Answer from the drawing. Dimensions are ordinates in mm from the lowest x, y and z of the part. A direction names the side the tool comes from. Coordinates: 2 decimals unless noted, no trailing zeros. Write each loop counter-clockwise with the first axis right and the second up, starting at its lowest first coordinate (ties: lowest second). Pieces come first, ordered by that corner, then holes.
(1) The part is cut by section B-B, the plane y = 10. Determine the outline of the cut face in (x, z), and give its area (3 significant figures).
(2) The part is cut by section D-D, the plane y = 17. Determine the outline of the cut face in (x, z), and give its area (3 significant figures).
(3) Which of the six approach directions +Z, -Z, +X, -X, +Y, -Y give full straight-line access (tool end or side, diameter ignored) to the marked faces 5, 6, 7 and 8?
(4) Given pin 1 (1.5 mm diameter, centred on y = 7, z = 6.5, fed in from +X); pin 2 (2.5 mm diameter, centred on x = 4, y = 6.5, fed in from +Z); pin 3 (5.5 mm diameter, centred on x = 17.5, y = 13.5, fed in from -Z), each flat-ended and moving along its own axis, determine where each tip first touches the part or whether it passes through.
(5) The part is cut by section C-C, the plane x = 37. Determine the outline of the cut face in (y, z).
(6) Straight lines are drawn through the part: line 1 along X through (y, z) = (10, 2.25); line 2 along X through (y, z) = (8.5, 8.75); line 3 along Y through (x, z) = (4, 2.15). For each, find the intervals that lie inside material, in ascending order.
(7) Determine the mould class of the marked faces 1, 2, 3 and 4 for opening direction X: pulls with the +X half, pulls with the -X half, needs draft (parallel to the pull), parting line crosses it, or undercut.
(8) The part is cut by section A-A, the plane z = 8. Determine the outline of the cut face in (x, y).
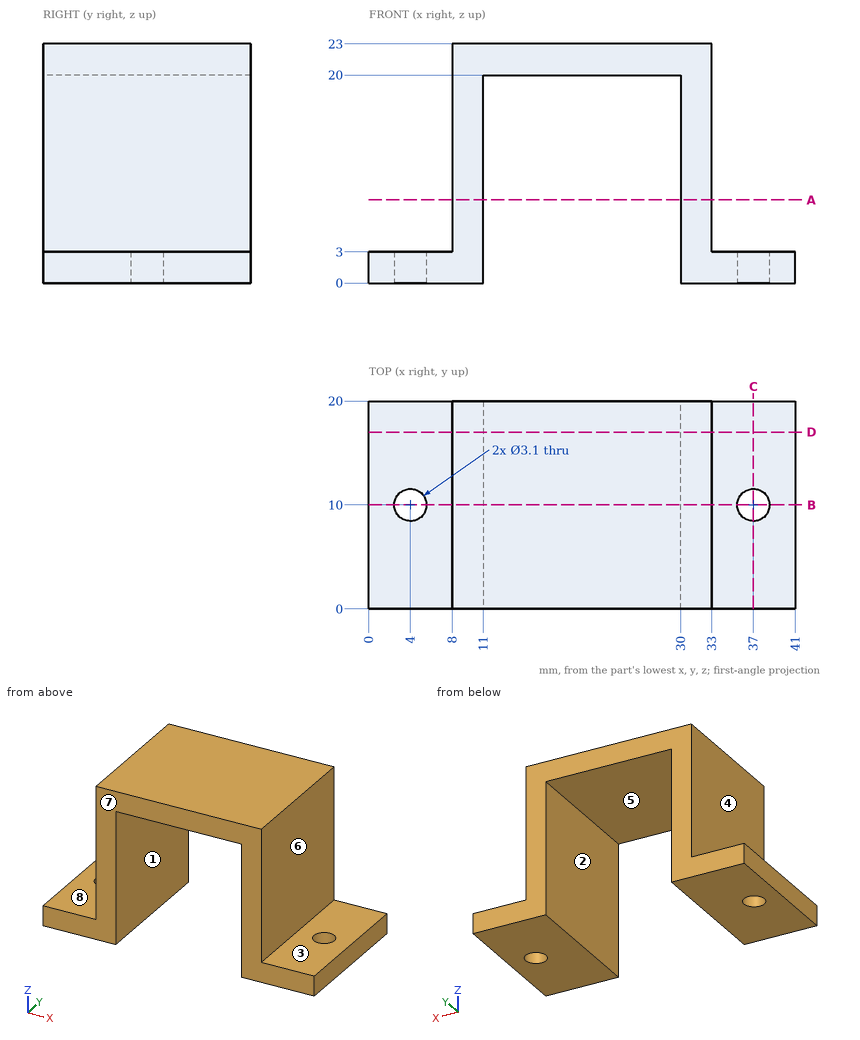
Computed:
1. outline: (0, 0) - (2.45, 0) - (2.45, 3) - (0, 3) - close; (5.55, 0) - (11, 0) - (11, 20) - (30, 20) - (30, 0) - (35.45, 0) - (35.45, 3) - (33, 3) - (33, 23) - (8, 23) - (8, 3) - (5.55, 3) - close; (38.55, 0) - (41, 0) - (41, 3) - (38.55, 3) - close
1. area: 224 mm2
2. outline: (0, 0) - (11, 0) - (11, 20) - (30, 20) - (30, 0) - (41, 0) - (41, 3) - (33, 3) - (33, 23) - (8, 23) - (8, 3) - (0, 3) - close
2. area: 243 mm2
3. face 5: -Z, +Y, -Y
3. face 6: +Z, +X, +Y, -Y
3. face 7: +Z, -Z, +X, -X, -Y
3. face 8: +Z, -X, +Y, -Y
4. pin 1: stops at x = 33
4. pin 2: stops at z = 3
4. pin 3: stops at z = 20
5. outline: (0, 0) - (8.45, 0) - (8.45, 3) - (0, 3) - close; (11.55, 0) - (20, 0) - (20, 3) - (11.55, 3) - close
6. line 1: x = 0 to 2.45, 5.55 to 11, 30 to 35.45, 38.55 to 41
6. line 2: x = 8 to 11, 30 to 33
6. line 3: y = 0 to 8.45, 11.55 to 20
7. face 1: undercut
7. face 2: undercut
7. face 3: needs draft
7. face 4: pulls with the -X half
8. outline: (8, 0) - (11, 0) - (11, 20) - (8, 20) - close; (30, 0) - (33, 0) - (33, 20) - (30, 20) - close
